Geometry check sheet. Reference: the model listing, model coordinates, mm. Coordinates: 2 decimals unless noted, no trailing zeros. Write each loop counter-clockwise with the first axis right and the second up, starting at its lowest first coordinate (ties: lowest second). Pieces come first, ordered by that corner, then holes. Notation, with made-up numbers: (27, -8) -> (84, -8) arc R16 ccw to (84, 8) -> close; hole circle Ø7 at (19, 2). An arc over 180 degrees is marked (long way). Answer in a Markdown table with one row per item. Add a question column.
Q1. Release check for a two-part mould opening along Y. For faces 1 (the face through (-49.469, -98, 15)), 2 (the face through (-43.454, 16.554, 15.21)), 3 (the face through (-149.469, -331, 15)) record: pulls with the +Y half, pulls with the -Y half, needs draft (parallel to the pull), parting line crosses it, or undercut.
Q2. Section check C-C, the plane y = -395. Record the boundary of the cut face in (x, z), and give its area (3 significant figures).
Q3. Thickness scan on line 1 (Y direction, x = 500, z = 11.75); line 2 (Y direction, x = 508, z = 13); line 3 (X direction, y = -115, z = 13.25). Record the ranges inside material, lowest first.
Q4. Gauge pin test, flat ends, axial feed: P1, Ø5, axis at y = -87, z = 15.5, coming from the +X side; P2, Ø7.5, axis at y = -87.5, z = 16.5, coming from the -X side; P3, Ø15, axis at y = -113, z = 10, coming from the -X side; P4, Ø12, axis at x = 279, y = -506.5, coming from the -Z side. Record the tip position at first contact, or that the pin passes through.
Q5. Section check B-B, the plane y = -499.5. Record the boundary of the cut face in (x, z), and give its area (3 significant figures).
Q6. Section check A-A, the plane z = 24.75. Record the boundary of the cut face in (x, y).
```python
from build123d import *

# Parameters (mm, degrees)
ESTRUSIONE_ESTRUSIONE2_DEPTH = 30
SCHIZZO3D1_R                 = 4.75
ESTRUSIONE_ESTRUSIONE7_DEPTH = 65
SCHIZZO3D1_5_R               = 4.75
ESTRUSIONE_ESTRUSIONE8_DEPTH = 65
RACCORDO3_R                  = 20
RACCORDO4_R                  = 20
RACCORDO5_R                  = 20
RACCORDO6_R                  = 20


with BuildPart() as part:
    # Schizzo1 → Estrusione-Estrusione2 (new body)
    with BuildSketch(Plane.XY):
        with BuildLine():
            Line((-49.46854998, 22.257563415), (450.53145002, 22.257563415))
            Line((450.53145002, 22.257563415), (450.53145002, -196.304936585))
            ThreePointArc((450.53145002, -196.304936585), (480.066711204, -266.421864704), (550.53145002, -295.117436585))
            Line((550.53145002, -295.117436585), (550.53145002, -365.117436585))
            ThreePointArc((550.53145002, -365.117436585), (480.066711204, -393.813008466), (450.53145002, -463.929936585))
            Line((450.53145002, -463.929936585), (450.53145002, -677.742436585))
            Line((450.53145002, -677.742436585), (-49.46854998, -677.742436585))
            Line((-49.46854998, -677.742436585), (-49.46854998, -463.929936585))
            ThreePointArc((-49.46854998, -463.929936585), (-79.003811164, -393.813008466), (-149.46854998, -365.117436585))
            Line((-149.46854998, -365.117436585), (-149.46854998, -295.117436585))
            ThreePointArc((-149.46854998, -295.117436585), (-79.003811164, -266.421864704), (-49.46854998, -196.304936585))
            Line((-49.46854998, -196.304936585), (-49.46854998, 22.257563415))
        make_face()
    extrude(amount=ESTRUSIONE_ESTRUSIONE2_DEPTH)

    # Schizzo3D1 → Estrusione-Estrusione7 (add)
    with BuildSketch(Plane(origin=(-114.46854998, -87.023686585, 15), x_dir=(0, -1, 0), z_dir=(-1, 0, 0))):
        with Locations(Location((0, 0, 0), (0, 0, 270))):
            Circle(SCHIZZO3D1_R)
        with Locations(Location((483.8125, 0, 0), (0, 0, 270))):
            Circle(SCHIZZO3D1_R)
    extrude(amount=-ESTRUSIONE_ESTRUSIONE7_DEPTH)

    # Schizzo3D1<5> → Estrusione-Estrusione8 (add)
    with BuildSketch(Plane(origin=(515.53145002, -87.023686585, 15), x_dir=(0, -1, 0), z_dir=(-1, 0, 0))):
        with Locations(Location((0, 0, 0), (0, 0, 270))):
            Circle(SCHIZZO3D1_5_R)
        with Locations(Location((483.8125, 0, 0), (0, 0, 270))):
            Circle(SCHIZZO3D1_5_R)
    extrude(amount=ESTRUSIONE_ESTRUSIONE8_DEPTH)

    # Raccordo3
    raccordo3_edges = [part.edges().sort_by_distance(p)[0] for p in [
        (-49.46854998, 22.257563415, 15),
    ]]
    fillet(raccordo3_edges, radius=RACCORDO3_R)

    # Raccordo4
    raccordo4_edges = [part.edges().sort_by_distance(p)[0] for p in [
        (450.53145002, 22.257563415, 15),
    ]]
    fillet(raccordo4_edges, radius=RACCORDO4_R)

    # Raccordo5
    raccordo5_edges = [part.edges().sort_by_distance(p)[0] for p in [
        (450.53145002, -677.742436585, 15),
    ]]
    fillet(raccordo5_edges, radius=RACCORDO5_R)

    # Raccordo6
    raccordo6_edges = [part.edges().sort_by_distance(p)[0] for p in [
        (-49.46854998, -677.742436585, 15),
    ]]
    fillet(raccordo6_edges, radius=RACCORDO6_R)


solid = part.part
```
Calculated:
| question | item | result |
|---|---|---|
| 1 | face 1 | undercut |
| 1 | face 2 | pulls with the +Y half |
| 1 | face 3 | needs draft |
| 2 | outline | (-77.82, 0) -> (478.89, 0) -> (478.89, 30) -> (-77.82, 30) -> close |
| 2 | area | 16,700 mm² |
| 3 | line 1 | y = -574.3 to -567.37, -378.57 to -281.67, -90.49 to -83.56 |
| 3 | line 2 | y = -575.14 to -566.53, -374.39 to -285.84, -91.33 to -82.72 |
| 3 | line 3 | x = -49.47 to 450.53 |
| 4 | P1 | stops at x = 515.53 |
| 4 | P2 | stops at x = -114.47 |
| 4 | P3 | stops at x = -49.47 |
| 4 | P4 | stops at z = 0 |
| 5 | outline | (-49.47, 0) -> (450.53, 0) -> (450.53, 30) -> (-49.47, 30) -> close |
| 5 | area | 15,000 mm² |
| 6 | outline | (-149.47, -365.12) arc R99.41 cw to (-49.47, -463.93) -> (-49.47, -657.74) arc R20 ccw to (-29.47, -677.74) -> (430.53, -677.74) arc R20 ccw to (450.53, -657.74) -> (450.53, -463.93) arc R99.41 cw to (550.53, -365.12) -> (550.53, -295.12) arc R99.41 cw to (450.53, -196.3) -> (450.53, 2.26) arc R20 ccw to (430.53, 22.26) -> (-29.47, 22.26) arc R20 ccw to (-49.47, 2.26) -> (-49.47, -196.3) arc R99.41 cw to (-149.47, -295.12) -> close |
